Part model, mm, in its own coordinate system. Face numbers are marked on the shaded views. Give positions to 0.01 mm unless a question says otherwise; leave off trailing zeros. Write item = value, one per line. Start each with the question number.
Item 1: Pull direction X, two halves, no side cores. Call the marked faces 1, 2 and 3: +X half, -X half, draft (parallel to the pull), parting line (faces both ways), or undercut.
Item 2: Drill centre lines: line 1 along Z through (x, y) = (-1.25, 13.25); line 2 along X through (y, z) = (12.25, -2.25); line 3 along X through (y, z) = (10.5, -2.5). Where is each one in solid material? Low to high.
Item 3: Flat gauge pins, fed straight in: P1, Ø1, axis at y = 7.5, z = -3.5, coming from the +X side; P2, Ø2, axis at y = 12, z = -3, coming from the -X side; P3, Ø2, axis at x = -2.5, y = 7, coming from the +Z side. Where does each tip first touch, or does it go through?
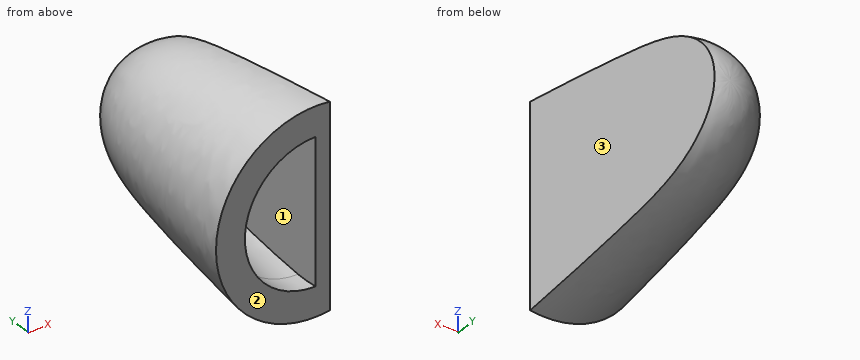
```python
from build123d import *

# Parameters (mm, degrees)
SKETCH5_W                = 5
SKETCH5_H                = 18
CUT_EXTRUDE4_DEPTH       = 20
REVOLVE3_ANGLE           = 90
REVOLVE3_OTHER_WAY_ANGLE = 90
SKETCH12_W               = 15.157920946
SKETCH12_H               = 18.962900337
CUT_EXTRUDE5_DEPTH       = 9


with BuildPart() as part:
    # Sketch1 → Revolve1 (revolve)
    with BuildSketch(Plane.XY):
        with BuildLine():
            Line((4.88, 0), (6.88, 0))
            add(Edge.make_bspline(
                [(6.88, 0), (6.476901655, 3.177692832), (5.808868292, 8.357754247), (4.378289276, 15.464596201), (1.111060579, 17.280233516), (0, 17.2)],
                knots=[0, 0, 0, 0, 0.473754928, 0.838492431, 1, 1, 1, 1], degree=3))
            Line((0, 17.2), (0, 15.4))
            add(Edge.make_bspline(
                [(0, 15.4), (1.563029619, 15.297760208), (2.284243197, 13.63319745)],
                knots=[0, 0, 0, 1, 1, 1], degree=2))
            add(Edge.make_bspline(
                [(2.284243197, 13.63319745), (4.266259497, 7.778351244), (4.88, 1.606249126)],
                knots=[0, 0, 0, 1, 1, 1], degree=2))
            ThreePointArc((4.88, 1.606249126), (4.905839008, 0.803124563), (4.88, 0))
        make_face()
    revolve(axis=Axis((0, 18.057905706, 0), (0, -1, 0)))

    # Sketch5 → Cut-Extrude4 (cut)
    with BuildSketch(Plane.XZ):
        with Locations((4.5, 0.912005105)):
            Rectangle(SKETCH5_W, SKETCH5_H)
    extrude(amount=-CUT_EXTRUDE4_DEPTH, mode=Mode.SUBTRACT)

    # Sketch9 → Revolve3 (revolve)
    with BuildSketch(Plane.XY):
        with BuildLine():
            Line((0, 17.2), (0, 0))
            Line((0, 0), (4.88, 0))
            Line((4.88, 0), (6.88, 0))
            add(Edge.make_bspline(
                [(6.88, 0), (6.476901655, 3.177692832), (5.808868292, 8.357754247), (4.378289276, 15.464596201), (1.111060579, 17.280233516), (0, 17.2)],
                knots=[0, 0, 0, 0, 0.473754928, 0.838492431, 1, 1, 1, 1], degree=3))
        make_face()
    revolve(axis=Axis((0, 17.2, 0), (0, -1, 0)), revolution_arc=REVOLVE3_ANGLE)

    # Sketch9 → Revolve3 other way (revolve)
    with BuildSketch(Plane.XY):
        with BuildLine():
            Line((0, 17.2), (0, 0))
            Line((0, 0), (4.88, 0))
            Line((4.88, 0), (6.88, 0))
            add(Edge.make_bspline(
                [(6.88, 0), (6.476901655, 3.177692832), (5.808868292, 8.357754247), (4.378289276, 15.464596201), (1.111060579, 17.280233516), (0, 17.2)],
                knots=[0, 0, 0, 0, 0.473754928, 0.838492431, 1, 1, 1, 1], degree=3))
        make_face()
    revolve(axis=Axis((0, 17.2, 0), (0, 1, 0)), revolution_arc=REVOLVE3_OTHER_WAY_ANGLE)

    # Sketch12 → Cut-Extrude5 (cut)
    with BuildSketch(Plane(origin=(10, 0, 0), x_dir=(0, 0, -1), z_dir=(1, 0, 0))):
        with Locations((0, 8.631516603)):
            Rectangle(SKETCH12_W, SKETCH12_H)
    extrude(amount=-CUT_EXTRUDE5_DEPTH, mode=Mode.SUBTRACT)


solid = part.part
```
Values found:
q1.face_1 = undercut
q1.face_2 = draft
q1.face_3 = +X half
q2.line_1 = -4.42 to -2.06, 2.06 to 4.42
q2.line_2 = -4.37 to -1.55, 0 to 1
q2.line_3 = -4.71 to -2.06, 0 to 1
q3.P1 = 1
q3.P2 = -4.65
q3.P3 = 5.77
